Source: CAD feature listing. Evaluate the final solid. Frame: model axes, mm. Coordinates: 2 decimals unless noted, no trailing zeros. Loops run counter-clockwise (first coordinate to the right, second up) from the corner with the lowest first, then second, coordinate; pieces in that order, holes last.
Item 1: Section query C-C, the plane x = 1. Return the cut outline in (y, z), then the cut area to 3 significant figures.
Item 2: Section query A-A, the plane y = -3.5. Return the cut outline in (x, z), then the cut area to 3 significant figures.
Item 3: Line query: probe 1 along Z at (x, y) = (5, -1.75); probe 2 along Z at (x, y) = (3, 3). Output: solid intervals per line, ascending.
Item 4: Section query B-B, the plane x = 8. Return the cut outline in (y, z).
```python
from build123d import *

# Parameters (mm, degrees)
F1_DEPTH = 4.6
F2_R     = 2


with BuildPart() as f1:
    # F0 (on Front) → F1 (new body, symmetric)
    with BuildSketch(Plane.XZ):
        Polygon((0, 5.25), (0, 0), (10, 0), (10, 5.25), (9.449296, 5.25), (7, 3.835898), (5, 2.681198), (3, 3.835898), (0.550704, 5.25), align=None)
    extrude(amount=F1_DEPTH, both=True)

    # F2
    f2_edges = [f1.edges().sort_by_distance(p)[0] for p in [
        (5, 0, 2.681198),
    ]]
    fillet(f2_edges, radius=F2_R)


solid = f1.part
```
Verdict:
1. outline: (-4.6, 0) - (4.6, 0) - (4.6, 4.99) - (-4.6, 4.99) - close
1. area: 45.9 mm2
2. outline: (0, 0) - (10, 0) - (10, 5.25) - (9.45, 5.25) - (7, 3.84) - (6, 3.26) arc R2 cw to (4, 3.26) - (3, 3.84) - (0.55, 5.25) - (0, 5.25) - close
2. area: 41.3 mm2
3. probe 1: z = 0 to 2.99
3. probe 2: z = 0 to 3.84
4. outline: (-4.6, 0) - (4.6, 0) - (4.6, 4.41) - (-4.6, 4.41) - close
